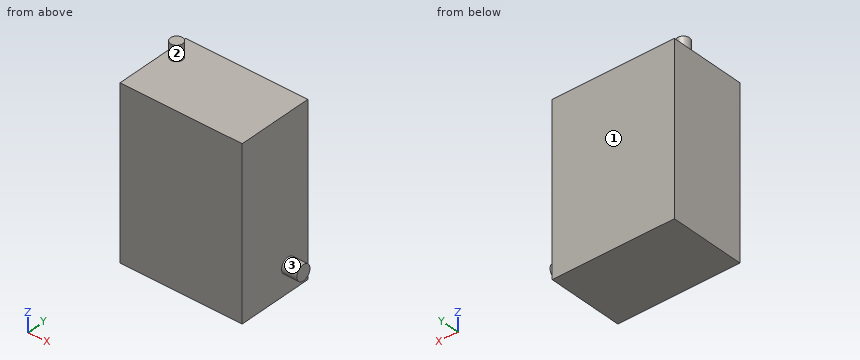
```python
from build123d import *

# Parameters (mm, degrees)
SKETCH1_W           = 110
SKETCH1_H           = 50
BOSS_EXTRUDE1_DEPTH = 80
SKETCH2_R           = 4
BOSS_EXTRUDE2_DEPTH = 10
SKETCH3_R           = 5
BOSS_EXTRUDE3_DEPTH = 10


with BuildPart() as part:
    # Sketch1 → Boss-Extrude1 (new body)
    with BuildSketch(Plane(origin=(0, 0, 0), x_dir=(0, 0, -1), z_dir=(1, 0, 0))):
        with Locations((55, 25)):
            Rectangle(SKETCH1_W, SKETCH1_H)
    extrude(amount=BOSS_EXTRUDE1_DEPTH)

    # Sketch2 → Boss-Extrude2 (add)
    with BuildSketch(Plane.XY):
        with Locations((7, 35)):
            Circle(SKETCH2_R)
    extrude(amount=BOSS_EXTRUDE2_DEPTH)

    # Sketch3 → Boss-Extrude3 (add)
    with BuildSketch(Plane(origin=(80, 0, 0), x_dir=(0, 0, -1), z_dir=(1, 0, 0))):
        with Locations((93, 35)):
            Circle(SKETCH3_R)
    extrude(amount=BOSS_EXTRUDE3_DEPTH)


solid = part.part
```
Verification items for the finished model (mm, model axes). Face numbers are marked on the shaded views. A direction names the side the tool comes from. Give positions to 0.01 mm unless a question says otherwise; leave off trailing zeros. Order: outer loops, then holes, each group sorted by start corner. A loop starts at its lowest first (then second) coordinate and runs counter-clockwise, first axis right, second up. Notation, with made-up numbers: (63, -8.75) -> (109, -8.75) arc R13 ccw to (109, 13.25) -> close; hole circle Ø10 at (9, 82). An arc over 180 degrees is marked (long way). Use a Markdown table: item, result.
1) Section check C-C, the plane x = 7. Record the boundary of the cut face in (y, z), then the cut area to 3 significant figures.
Results:
| item | result |
|---|---|
| outline | (0, -110) -> (50, -110) -> (50, 0) -> (39, 0) -> (39, 10) -> (31, 10) -> (31, 0) -> (0, 0) -> close |
| area | 5,580 mm² |
2) Depth check by flat-ended pin: pin 1 Ø1 at (x, y) = (64.5, 10) entering from +Z; pin 2 Ø15 at (y, z) = (16.5, -41.5) entering from +X. Enter the tip coordinate at first touch or a pass-through.
Results:
| item | result |
|---|---|
| pin 1 | z = 0 |
| pin 2 | x = 80 |
3) Section check D-D, the plane y = 16.5. Record the boundary of the cut face in (x, z), then the cut area to 3 significant figures.
Results:
| item | result |
|---|---|
| outline | (0, -110) -> (80, -110) -> (80, 0) -> (0, 0) -> close |
| area | 8,800 mm² |
4) Section check B-B, the plane z = -93. Record the boundary of the cut face in (x, y), then the cut area to 3 significant figures.
Results:
| item | result |
|---|---|
| outline | (0, 0) -> (80, 0) -> (80, 30) -> (90, 30) -> (90, 40) -> (80, 40) -> (80, 50) -> (0, 50) -> close |
| area | 4,100 mm² |
5) Material ranges on probe 1 along X at (y, z) = (32.5, -35); probe 2 along Z at (x, y) = (56.5, 9.5), recorded low to high.
Results:
| item | result |
|---|---|
| probe 1 | 0 to 80 |
| probe 2 | -110 to 0 |
6) Tool access check on the marked faces 1, 2 and 3. Record the directions out of +Z, -Z, +X, -X, +Y, -Y that give a thin tool (end or side, any length) a straight path to the whole face; none if there is none.
Results:
| item | result |
|---|---|
| face 1 | +Z, -Z, +X, -X, +Y |
| face 2 | +Z |
| face 3 | +X |
7) Section check A-A, the plane y = 35. Record the boundary of the cut face in (x, z).
Results:
| item | result |
|---|---|
| outline | (0, -110) -> (80, -110) -> (80, -98) -> (90, -98) -> (90, -88) -> (80, -88) -> (80, 0) -> (11, 0) -> (11, 10) -> (3, 10) -> (3, 0) -> (0, 0) -> close |
